from build123d import *

# Parameters (mm, degrees)
SKETCH_1_R      = 2
EXTRUDE_1_DEPTH = 1.5


with BuildPart() as part:
    # 草图1 → 凸台-拉伸1 (new, symmetric)
    with BuildSketch(Plane.XY):
        with BuildLine():
            ThreePointArc((52.051282327, 4.604617186), (27.130077256, 0.338946041), (2.190311245, 4.494723201))
            ThreePointArc((2.190311245, 4.494723201), (1.655516013, 4.681596435), (1.122130296, 4.872455603))
            ThreePointArc((1.122130296, 4.872455603), (-4.395154703, 2.383823638), (-3.472004537, -3.597941702))
            ThreePointArc((-3.472004537, -3.597941702), (1.030595655, -14.252623677), (3.610487783, -25.528252843))
            ThreePointArc((3.610487783, -25.528252843), (9.300815316, -32.038345872), (17.342543053, -28.861593809))
            ThreePointArc((17.342543053, -28.861593809), (17.509155318, -28.5792742), (17.677657577, -28.298078543))
            ThreePointArc((17.677657577, -28.298078543), (33.128101274, -12.422940849), (54, -5))
            ThreePointArc((54, -5), (58.950668102, 0.700632103), (52.612561199, 4.803645863))
            ThreePointArc((52.612561199, 4.803645863), (52.332116942, 4.703581101), (52.051282327, 4.604617186))
        make_face()
        with Locations((11.07, -24.75)):
            Circle(SKETCH_1_R, mode=Mode.SUBTRACT)
        Circle(SKETCH_1_R, mode=Mode.SUBTRACT)
        with Locations((54, 0)):
            Circle(SKETCH_1_R, mode=Mode.SUBTRACT)
    extrude(amount=EXTRUDE_1_DEPTH, both=True)


solid = part.part
Can you work these out from the model? Positions are in its coordinate system, mm. Coordinates: 2 decimals unless noted, no trailing zeros. Loops run counter-clockwise (first coordinate to the right, second up) from the corner with the lowest first, then second, coordinate; pieces in that order, holes last. Notation, with made-up numbers: (-16.5, -15) - (-12.5, -15) arc R32 cw to (-12.5, 24) - close; hole circle Ø1 at (18, 88.25). An arc over 180 degrees is marked (long way). Put each result on its own line as item: value. Start each with the question number.
Item 1: Suppose I cut it at B-B (z = -0.8). Please give me the cut outline in (x, y), and give its area (3 significant figures).
Item 2: Suppose I cut it at D-D (y = -15.5). Please give me the cut outline in (x, z), and give its area (3 significant figures).
Item 3: If we mould it in two halves opening along X, with no side actions, what happens to faces 1 (the face through (19, -9, -1.5)), 2 (the face through (0.98, -14.1, 0.02)), 3 (the face through (52, 0, 0)), 4 (the face through (0, -2, 0))? For each: +X half, -X half, draft (parallel to the pull), parting line (faces both ways), or undercut.
Item 4: If I drill on line 1 along Y through (x, z) = (54, 0.35); line 2 along Y through (x, z) = (11.07, -0.15); line 3 along X through (y, z) = (-1, 1.35), over which ranges is the centre line in solid material (lowest first)?
Item 5: For pin 1 (1 mm diameter, centred on x = 13.5, z = -0.5, fed in from +Y), with a flat end and sliding along its axis, tell me the tip position at first contact or that it passes through.
Item 6: Suppose I cut it at A-A (y = -24.75). Please give me the cut outline in (x, z), and give its area (3 significant figures).
Item 7: Suppose I cut it at C-C (x = 11.07). Please give me the cut outline in (y, z).
Here are the results:
1. outline: (-3.47, -3.6) arc R66.22 cw to (3.61, -25.53) arc R7.5 ccw to (17.34, -28.86) arc R48.87 cw to (17.68, -28.3) arc R48.87 cw to (54, -5) arc R5 ccw (long way) to (52.61, 4.8) arc R75.91 cw to (52.05, 4.6) arc R75.91 cw to (2.19, 4.49) arc R75.91 cw to (1.12, 4.87) arc R5 ccw to start; hole circle Ø4 at (0, 0); hole circle Ø4 at (11.07, -24.75); hole circle Ø4 at (54, 0)
1. area: 1,110 mm²
2. outline: (1.42, -1.5) - (28.86, -1.5) - (28.86, 1.5) - (1.42, 1.5) - close
2. area: 82.3 mm²
3. face 1: draft
3. face 2: -X half
3. face 3: undercut
3. face 4: undercut
4. line 1: -5 to -2, 2 to 5
4. line 2: -32.25 to -26.75, -22.75 to 2.02
4. line 3: -4.9 to -1.73, 1.73 to 52.27, 55.73 to 58.9
5. pin 1: y = 1.63
6. outline: (3.5, -1.5) - (9.07, -1.5) - (9.07, 1.5) - (3.5, 1.5) - close; (13.07, -1.5) - (20.04, -1.5) - (20.04, 1.5) - (13.07, 1.5) - close
6. area: 37.6 mm²
7. outline: (-32.25, -1.5) - (-26.75, -1.5) - (-26.75, 1.5) - (-32.25, 1.5) - close; (-22.75, -1.5) - (2.02, -1.5) - (2.02, 1.5) - (-22.75, 1.5) - close
